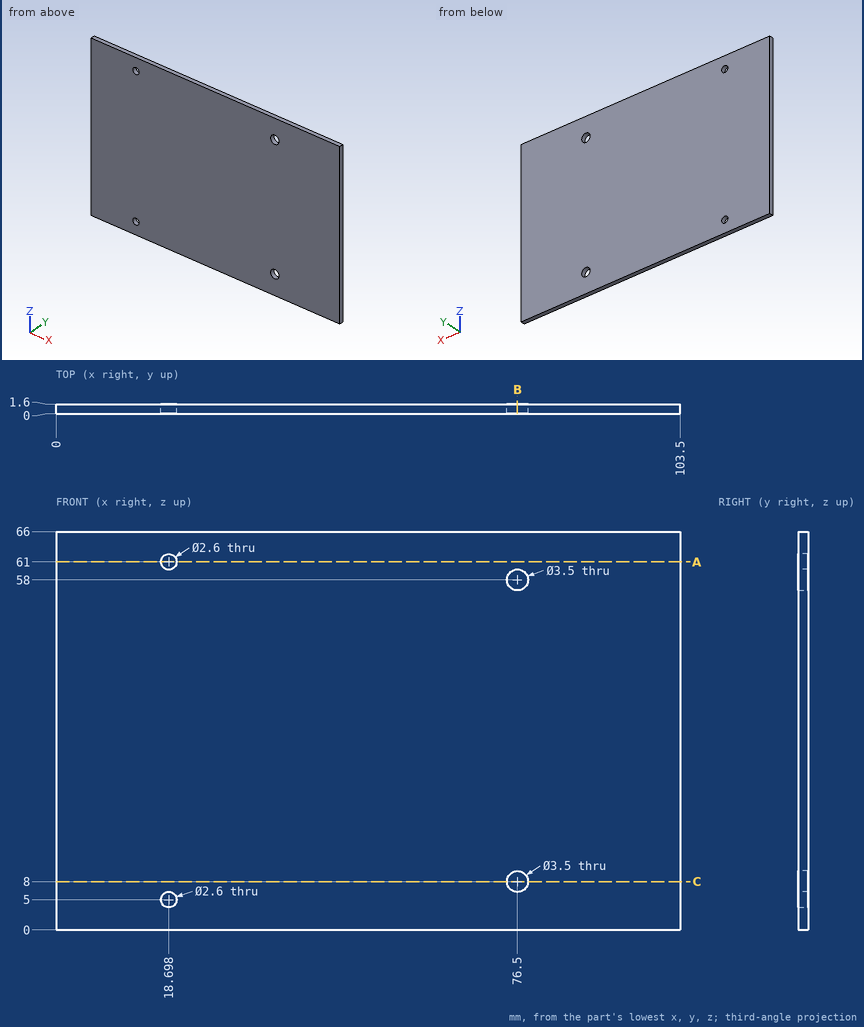
Print and shaded views of the part. All mm, measured from the part's lowest x, y and z. Round coordinates to 2 decimals unless told otherwise and drop trailing zeros. Write each loop counter-clockwise with the first axis right and the second up, starting at its lowest first coordinate (ties: lowest second). Pieces come first, ordered by that corner, then holes. Notation, with made-up numbers: (-17.75, -32.75) - (21.25, -32.75) arc R24 ccw to (21.25, -18.75) - close; hole circle Ø1 at (2.5, 33). An arc over 180 degrees is marked (long way). Write each question's results on one line, items separated by ' | '. Start each with the question number.
Item 1: Saw through at B-B (x = 76.5). Write the cut outline in (y, z).
Item 2: Wall check: L1, parallel to Z at x = 76.5, y = 1; L2, parallel to X at y = 1.15, z = 61; L3, parallel to X at y = 0.5, z = 58. Give the ranges that are in metal, low to high. Write a range as [from, to].
Item 3: Saw through at A-A (z = 61). Write the cut outline in (x, y).
Item 4: Saw through at C-C (z = 8). Write the cut outline in (x, y), and give its area (3 significant figures).
Results are:
1) outline: (0, 0) - (1.6, 0) - (1.6, 6.25) - (0, 6.25) - close; (0, 9.75) - (1.6, 9.75) - (1.6, 56.25) - (0, 56.25) - close; (0, 59.75) - (1.6, 59.75) - (1.6, 66) - (0, 66) - close
2) L1: z = [0, 6.25], [9.75, 56.25], [59.75, 66] | L2: x = [0, 17.4], [20, 103.5] | L3: x = [0, 74.75], [78.25, 103.5]
3) outline: (0, 0) - (17.4, 0) - (17.4, 1.6) - (0, 1.6) - close; (20, 0) - (103.5, 0) - (103.5, 1.6) - (20, 1.6) - close
4) outline: (0, 0) - (74.75, 0) - (74.75, 1.6) - (0, 1.6) - close; (78.25, 0) - (103.5, 0) - (103.5, 1.6) - (78.25, 1.6) - close | area: 160 mm²
